Input: part model. Units: mm. Frame: model coordinates. A direction names the side the tool comes from. Coordinates: 2 decimals unless noted, no trailing zeros. Order: outer loops, then holes, each group sorted by start corner. A loop starts at its lowest first (then second) coordinate and runs counter-clockwise, first axis right, second up.
from build123d import *

# Parameters (mm, degrees)
F1_DEPTH = 2


with BuildPart() as f1:
    # F0 (on Front) → F1 (new body)
    with BuildSketch(Plane.XZ):
        Polygon((-10, -14), (10, -14), (10, 14), (3.3, 14), (3.3, 12.5), (4, 12.5), (4, 4), (3, 0.5), (3, -5), (1, -5), (1, 0), (0, 0), (-1, 0), (-1, -5), (-3, -5), (-3, 0.5), (-4, 4), (-4, 12.5), (-3.3, 12.5), (-3.3, 14), (-10, 14), align=None)
    extrude(amount=F1_DEPTH)


solid = f1.part
Item 1: Cut plane A-A on z = 7.75. Return loops of the section in (x, y), then the cut area to 3 significant figures.
Response values:
outline: (-10, -2) - (-4, -2) - (-4, 0) - (-10, 0) - close; (4, -2) - (10, -2) - (10, 0) - (4, 0) - close
area: 24.0 mm2
Item 2: Access query for faces 4 (the face through (4, -1, 8)), 5 (the face through (3, -1, -2)), 6 (the face through (0, -2, -3)). Directions: +Z, -Z, +X, -X, +Y, -Y. A direction counts if a zero-diameter tool reaches every point of the face in a straight line with its end or side. Return the directions, or none.
Response values:
face 4: +Y, -Y
face 5: +Z, +Y, -Y
face 6: +Z, -Z, +X, -X, -Y
Item 3: Pin query (flat end, axial travel): pin 1 Ø0.6 at (x, y) = (1.5, -0.5) entering from +Z; pin 2 Ø3 at (x, z) = (-1.5, 9) entering from +Y; pin 3 Ø1.5 at (x, z) = (4, 3) entering from +Y. Return the tip coordinate at first contact, or that it passes through.
Response values:
pin 1: stops at z = -5
pin 2: passes through
pin 3: stops at y = 0
Item 4: Cut plane B-B on z = -0.5. Return loops of the section in (x, y), then the cut area to 3 significant figures.
Response values:
outline: (-10, -2) - (-3, -2) - (-3, 0) - (-10, 0) - close; (-1, -2) - (1, -2) - (1, 0) - (-1, 0) - close; (3, -2) - (10, -2) - (10, 0) - (3, 0) - close
area: 32.0 mm2
Item 5: Cut plane D-D on x = -0.5. Return loops of the section in (y, z).
Response values:
outline: (-2, -14) - (0, -14) - (0, 0) - (-2, 0) - close
Item 6: Draft query along X for faces 1 (the face through (-3, -1, -2)), 2 (the face through (0, 0, -3)), 3 (the face through (-10, -1, 0)). Return one class per face: pulls with the +X half, pulls with the -X half, needs draft (parallel to the pull), parting line crosses it, or undercut.
Response values:
face 1: undercut
face 2: needs draft
face 3: pulls with the -X half
Item 7: Cut plane C-C on y = -0.75. Return loops of the section in (x, z), then the cut area to 3 significant figures.
Response values:
outline: (-10, -14) - (10, -14) - (10, 14) - (3.3, 14) - (3.3, 12.5) - (4, 12.5) - (4, 4) - (3, 0.5) - (3, -5) - (1, -5) - (1, 0) - (-1, 0) - (-1, -5) - (-3, -5) - (-3, 0.5) - (-4, 4) - (-4, 12.5) - (-3.3, 12.5) - (-3.3, 14) - (-10, 14) - close
area: 435 mm2
Item 8: Ray query, probe 1 along X at (y, z) = (-0.75, 5); probe 2 along X at (y, z) = (-0.5, -3); probe 3 along Z at (x, y) = (-0.75, -1.15). Return the intervals inside material, ascending.
Response values:
probe 1: x = -10 to -4, 4 to 10
probe 2: x = -10 to -3, -1 to 1, 3 to 10
probe 3: z = -14 to 0
